```python
from build123d import *

# Parameters (mm, degrees)
F1_DEPTH      = 12.7
F6_DEPTH      = 511.1661396565
F6_DEPTH_BACK = 511.1661396565
F7_DEPTH      = 457.201


with BuildPart() as f1:
    # F0 (on Front) → F1 (new body)
    with BuildSketch(Plane.XZ):
        Polygon((0, -457.2), (0, 0), (-914.4, 0), align=None)
    extrude(amount=F1_DEPTH)

    # F5 (on face) → F6 (cut, two sides)
    with BuildSketch(Plane(origin=(-274.32, 0, 137.16), x_dir=(0, -1, 0), z_dir=(-0.894427191, 0, 0.4472135955))) as f6_sk:
        Polygon((12.7, -406.8387485734), (0, -408.9321117252), (12.7, -408.9321117252), align=None)
    extrude(amount=-F6_DEPTH, mode=Mode.SUBTRACT)
    extrude(f6_sk.sketch, amount=F6_DEPTH_BACK, mode=Mode.SUBTRACT)

    # F2 (on face) → F7 (cut, through all)
    with BuildSketch(Plane.XY):
        Polygon((-914.4, -12.7), (-808.223047, -12.7), (-812.7131750519, 0), (-914.4, 0), align=None)
        Polygon((-4.4901280519, 0), (0, -12.7), (0, 0), align=None)
    extrude(amount=-F7_DEPTH, mode=Mode.SUBTRACT)


solid = f1.part
```
The model under review builds one solid part; all positions refer to its coordinate system, in mm. Coordinates: 2 decimals unless noted, no trailing zeros. Write each loop counter-clockwise with the first axis right and the second up, starting at its lowest first coordinate (ties: lowest second). Pieces come first, ordered by that corner, then holes.
1) Clearance check with flat-ended pins moving along their axes: pin 1 Ø2 at (x, y) = (-467, -2) entering from -Z; pin 2 Ø1.5 at (y, z) = (-6.5, -105.5) entering from -X; pin 3 Ø6 at (y, z) = (-9, -65.5) entering from +X. State where each tip first meets the part, or that it passes through.
2) To check wall thickness, follow probe 1 along X at (y, z) = (-3.5, -404.5); probe 2 along X at (y, z) = (-8.75, -73); probe 3 along Z at (x, y) = (-210, -11.25). State the ranges of each line that lie inside material, in increasing order.
3) We need section B-B on x = -471.5. State the section outline as (y, z) points.
4) We need section A-A on z = -283. State the section outline as (x, y) points.
Answer list:
1. pin 1: stops at z = -223.86
1. pin 2: stops at x = -702.53
1. pin 3: stops at x = -0.25
2. probe 1: x = -104.11 to -3.25
2. probe 2: x = -765.17 to -1.4
2. probe 3: z = -350.13 to 0
3. outline: (-12.7, -219.11) - (0, -221.45) - (0, 0) - (-12.7, 0) - close
4. outline: (-348.4, 0) - (-343.72, -12.7) - (0, -12.7) - (-4.49, 0) - close
